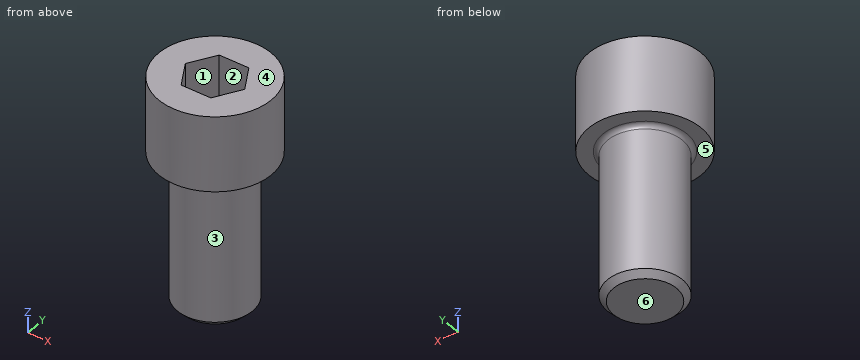
```python
from build123d import *

# Parameters (mm, degrees)
SKETCH1_W          = 1.875
SKETCH1_H          = 2.5
SKETCH1_W_2        = 1.25
SKETCH1_H_2        = 5
CUT_EXTRUDE1_DEPTH = 1.5
FILLET1_R          = 0.15
CHAMFER1_SIZE      = 0.2


with BuildPart() as part:
    # Sketch1 → Revolve1 (revolve)
    with BuildSketch(Plane(origin=(0, 0, 0), x_dir=(1, 0, 0), z_dir=(0, 1, 0))):
        with Locations((0.9375, 1.25)):
            Rectangle(SKETCH1_W, SKETCH1_H)
        with Locations((0.625, 5)):
            Rectangle(SKETCH1_W_2, SKETCH1_H_2)
    revolve(axis=Axis((0, 0, -2.5), (0, 0, -1)))

    # Sketch2 → Cut-Extrude1 (cut)
    with BuildSketch(Plane.XY):
        Polygon((1, 0), (0.5, 0.866025404), (-0.5, 0.866025404), (-1, 0), (-0.5, -0.866025404), (0.5, -0.866025404), align=None)
    extrude(amount=-CUT_EXTRUDE1_DEPTH, mode=Mode.SUBTRACT)

    # Fillet1
    fillet1_edges = [part.edges().sort_by_distance(p)[0] for p in [
        (-1.25, 0, -2.5),
    ]]
    fillet(fillet1_edges, radius=FILLET1_R)

    # Chamfer1
    chamfer1_edges = [part.edges().sort_by_distance(p)[0] for p in [
        (-1.25, 0, -7.5),
    ]]
    chamfer(chamfer1_edges, length=CHAMFER1_SIZE)


solid = part.part
```
CAD build for the part. Positions are in the model's coordinates, mm. Face numbers are marked on the shaded views. A direction names the side the tool comes from. Round coordinates to 2 decimals unless told otherwise and drop trailing zeros. Loops run counter-clockwise (first coordinate to the right, second up) from the corner with the lowest first, then second, coordinate; pieces in that order, holes last. Notation, with made-up numbers: M -9,70 L 49,70 A19 cw 49,102 Z; hole C -9.75,77.5 d2. An arc over 180 degrees is marked long. Return JSON: item names as keys, results as strings. Group by question number.
(1) Drop flat-ended pins along their axis: P1, Ø1, axis at y = -1, z = -4, coming from the +X side; P2, Ø2, axis at x = 1.5, z = -2.5, coming from the -Y side. Give the stop position or say it passes through.
(2) Saw through at A-A, the plane x = 0. List the corners of the cut face in (y, z) (3 decimals).
(3) Saw through at B-B, the plane z = -3.5. List the corners of the cut face in (x, y), and give its area (3 significant figures).
(4) Mould opens along X. For the marked faces 1, 2, 3 and 4 say: +X half, -X half, draft (parallel to the pull), parting line (faces both ways), or undercut.
(5) Tool access for the marked faces 5 and 6: list every direction of +Z, -Z, +X, -X, +Y, -Y with a clear straight run to the whole face (end or side of a thin tool).
(6) Wall check: probe 1 along Z at (x, y) = (0.7, -0.15); probe 2 along Z at (x, y) = (1.65, -0.35); probe 3 along X at (y, z) = (0.75, -3.75). Give the ranges that are in metal, low to high. Write a range as [from, to].
Answer list:
{
 "1": {"P1": "x = 1.15", "P2": "y = -1.81"},
 "2": {"outline": "M -1.875,-2.5 L -1.4,-2.5 A0.15 cw -1.25,-2.65 L -1.25,-7.3 L -1.05,-7.5 L 1.05,-7.5 L 1.25,-7.3 L 1.25,-2.65 A0.15 cw 1.4,-2.5 L 1.875,-2.5 L 1.875,0 L 0.866,0 L 0.866,-1.5 L -0.866,-1.5 L -0.866,0 L -1.875,0 Z"},
 "3": {"outline": "C 0,0 d2.5", "area": "4.91 mm2"},
 "4": {"face 1": "undercut", "face 2": "undercut", "face 3": "parting line", "face 4": "draft"},
 "5": {"face 5": "-Z", "face 6": "-Z, +X, -X, +Y, -Y"},
 "6": {"probe 1": "[-7.5, -1.5]", "probe 2": "[-2.5, 0]", "probe 3": "[-1, 1]"}
}
